Check sheet for the drawn part. Datum: minimum x, y, z corner. Units: mm. Round coordinates to 2 decimals unless told otherwise and drop trailing zeros. Write each loop counter-clockwise with the first axis right and the second up, starting at its lowest first coordinate (ties: lowest second). Pieces come first, ordered by that corner, then holes. Notation, with made-up numbers: (77.25, -30.5) - (103.25, -30.5) arc R35 ccw to (103.25, 5.5) - close; hole circle Ø7 at (3, -33.5). An arc over 180 degrees is marked (long way). Answer as a JSON object with one key per item and string values. Group by question number.
Item 1: Gauge pin test, flat end, axial feed: P1, Ø0.8, axis at x = 12, z = 1, coming from the +Y side. Record the tip position at first contact, or that the pin passes through.
Item 2: Thickness scan on line 1 (Y direction, x = 9.5, z = 0.45); line 2 (X direction, y = 1.8, z = 1.3); line 3 (X direction, y = 1.8, z = 0.8). Record the ranges inside material, lowest first.
Item 3: Sectioned sample at D-D on x = 5.75. Record the boundary of the cut face in (y, z).
Item 4: Sectioned sample at A-A on y = 1.8. Record the boundary of the cut face in (x, z).
Item 5: Sectioned sample at B-B on x = 9.5. Record the boundary of the cut face in (y, z).
Item 6: Release check for a two-part mould opening along Y. For the marked faces 1, 2 and 3 record: pulls with the +Y half, pulls with the -Y half, needs draft (parallel to the pull), parting line crosses it, or undercut.
Item 7: Sectioned sample at C-C on z = 1.4. Record the boundary of the cut face in (x, y), plus the area to 3 significant figures.
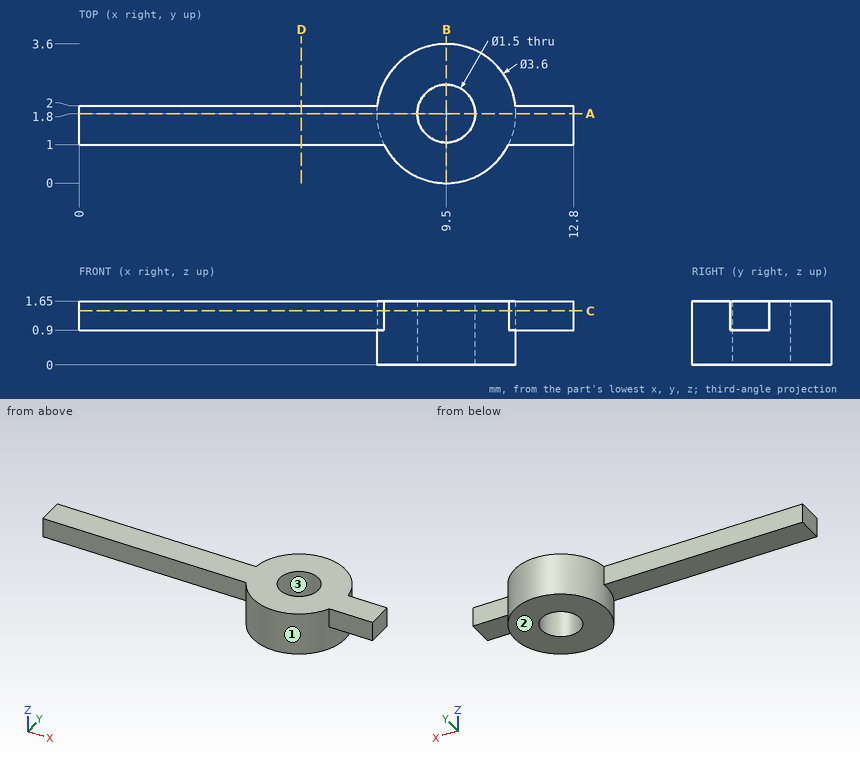
Completed:
{
 "1": {"P1": "y = 2"},
 "2": {"line 1": "0 to 1.05, 2.55 to 3.6", "line 2": "0 to 8.75, 10.25 to 12.8", "line 3": "7.7 to 8.75, 10.25 to 11.3"},
 "3": {"outline": "(1, 0.9) - (2, 0.9) - (2, 1.65) - (1, 1.65) - close"},
 "4": {"outline": "(0, 0.9) - (7.7, 0.9) - (7.7, 0) - (8.75, 0) - (8.75, 1.65) - (0, 1.65) - close; (10.25, 0) - (11.3, 0) - (11.3, 0.9) - (12.8, 0.9) - (12.8, 1.65) - (10.25, 1.65) - close"},
 "5": {"outline": "(0, 0) - (1.05, 0) - (1.05, 1.65) - (0, 1.65) - close; (2.55, 0) - (3.6, 0) - (3.6, 1.65) - (2.55, 1.65) - close"},
 "6": {"face 1": "parting line crosses it", "face 2": "needs draft", "face 3": "undercut"},
 "7": {"outline": "(0, 1) - (7.89, 1) arc R1.8 ccw to (11.11, 1) - (12.8, 1) - (12.8, 2) - (11.29, 2) arc R1.8 ccw to (7.71, 2) - (0, 2) - close; hole circle Ø1.5 at (9.5, 1.8)", "area": "17.7 mm²"}
}
